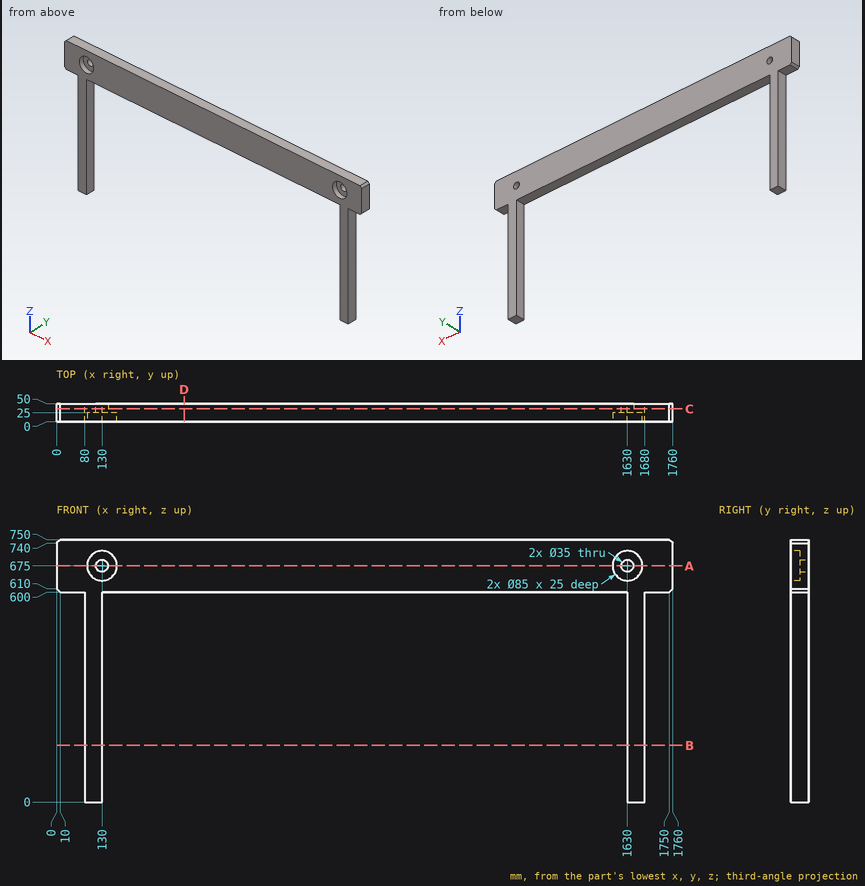
Job drawing, mm, ordinate dimensions from the low corner. One solid piece. Give positions to 0.01 mm unless a question says otherwise; leave off trailing zeros. Order: outer loops, then holes, each group sorted by start corner. A loop starts at its lowest first (then second) coordinate and runs counter-clockwise, first axis right, second up. Notation, with made-up numbers: (36, 23.25) -> (40, 23.25) arc R25 cw to (40, 48.25) -> close; hole circle Ø10 at (-2, 76.25). An arc over 180 degrees is marked (long way). Return JSON: item names as keys, results as strings.
Q1. Saw through at C-C (y = 36). Write the cut outline in (x, z), then the cut area to 3 significant figures.
Working result:
{"outline": "(0, 610) -> (10, 600) -> (80, 600) -> (80, 0) -> (130, 0) -> (130, 600) -> (1630, 600) -> (1630, 0) -> (1680, 0) -> (1680, 600) -> (1750, 600) -> (1760, 610) -> (1760, 740) -> (1750, 750) -> (10, 750) -> (0, 740) -> close; hole circle Ø35 at (130, 675); hole circle Ø35 at (1630, 675)", "area": "322,000 mm²"}
Q2. Flat gauge pins, fed straight in: pin 1 (15 mm diameter, centred on y = 27, z = 179.5, fed in from -X); pin 2 (25 mm diameter, centred on x = 48, y = 23, fed in from -Z); pin 3 (6 mm diameter, centred on y = 33, z = 550, fed in from +X). Where does each tip first touch, or does it go through?
Working result:
{"pin 1": "x = 80", "pin 2": "z = 600", "pin 3": "x = 1680"}
Q3. Saw through at A-A (z = 675). Write the cut outline in (x, y).
Working result:
{"outline": "(0, 0) -> (87.5, 0) -> (87.5, 25) -> (112.5, 25) -> (112.5, 50) -> (0, 50) -> close; (147.5, 25) -> (172.5, 25) -> (172.5, 0) -> (1587.5, 0) -> (1587.5, 25) -> (1612.5, 25) -> (1612.5, 50) -> (147.5, 50) -> close; (1647.5, 25) -> (1672.5, 25) -> (1672.5, 0) -> (1760, 0) -> (1760, 50) -> (1647.5, 50) -> close"}
Q4. Saw through at D-D (x = 364). Write the cut outline in (y, z).
Working result:
{"outline": "(0, 600) -> (50, 600) -> (50, 750) -> (0, 750) -> close"}
Q5. Drill centre lines: line 1 (X direction, y = 31, z = 675); line 2 (X direction, y = 21, z = 152); line 3 (X direction, y = 35.5, z = 682). Where is each one in solid material? Low to high.
Working result:
{"line 1": "0 to 112.5, 147.5 to 1612.5, 1647.5 to 1760", "line 2": "80 to 130, 1630 to 1680", "line 3": "0 to 113.96, 146.04 to 1613.96, 1646.04 to 1760"}
Q6. Saw through at B-B (z = 162.5). Write the cut outline in (x, y), then the cut area to 3 significant figures.
Working result:
{"outline": "(80, 0) -> (130, 0) -> (130, 50) -> (80, 50) -> close; (1630, 0) -> (1680, 0) -> (1680, 50) -> (1630, 50) -> close", "area": "5,000 mm²"}
